Check sheet for the modelled part. Datum: model origin and axes. Units: mm. Face numbers are marked on the shaded views. A direction names the side the tool comes from. Round coordinates to 2 decimals unless told otherwise and drop trailing zeros. Order: outer loops, then holes, each group sorted by start corner. A loop starts at its lowest first (then second) coordinate and runs counter-clockwise, first axis right, second up.
```python
from build123d import *

# Parameters (mm, degrees)
F0_R     = 4.75
F1_DEPTH = 2
F2_W     = 1
F2_H     = 0.5
F3_W     = 1
F3_H     = 0.5
F4_DEPTH = 2.5
F5_R     = 0.49999
F6_R     = 0.99999


# Not quite as in the source:
# - a fillet or chamfer is up to 0.001 mm smaller than in the source, because OpenCascade refuses the exact size


with BuildPart() as f1:
    # F0 (on Top) → F1 (new body)
    with BuildSketch(Plane.XY):
        Circle(F0_R)
        with BuildLine():
            ThreePointArc((-2.6457513111, 0.75), (0, 2.75), (2.6457513111, 0.75))
            Line((2.6457513111, 0.75), (3.6457513111, 0.75))
            Line((3.6457513111, 0.75), (3.6457513111, -0.75))
            Line((3.6457513111, -0.75), (2.6457513111, -0.75))
            ThreePointArc((2.6457513111, -0.75), (0, -2.75), (-2.6457513111, -0.75))
            Line((-2.6457513111, -0.75), (-3.6457513111, -0.75))
            Line((-3.6457513111, -0.75), (-3.6457513111, 0.75))
            Line((-3.6457513111, 0.75), (-2.6457513111, 0.75))
        make_face(mode=Mode.SUBTRACT)
    extrude(amount=F1_DEPTH)

    # F2 (on face) + F3 (on face) → F4 (join)
    with BuildSketch(Plane.XZ.offset(-0.75)):
        with Locations((-3.1457513111, 1.75)):
            Rectangle(F2_W, F2_H)
        with Locations((-3.1457513111, 0.25)):
            Rectangle(F2_W, F2_H)
    with BuildSketch(Plane.XZ.offset(-0.75)):
        with Locations((3.1457513111, 0.25)):
            Rectangle(F3_W, F3_H)
        with Locations((3.1457513111, 1.75)):
            Rectangle(F3_W, F3_H)
    extrude(amount=F4_DEPTH)

    # F5 (radius 0.5 in the source; OpenCascade refuses exactly that, so slightly less here)
    f5_edges = [f1.edges().sort_by_distance(p)[0] for p in [
        (-2.645751, 0, 2),
        (2.645751, 0, 2),
        (0, 2.75, 2),
        (0, -2.75, 2),
        (0, 2.75, 0),
        (0, -2.75, 0),
        (-2.645751, 0, 0),
        (2.645751, 0, 0),
    ]]
    fillet(f5_edges, radius=F5_R)

    # F6 (radius 1 in the source; OpenCascade refuses exactly that, so slightly less here)
    f6_edges = [f1.edges().sort_by_distance(p)[0] for p in [
        (-4.75, 0, 2),
        (-4.75, 0, 0),
    ]]
    fillet(f6_edges, radius=F6_R)


solid = f1.part
```
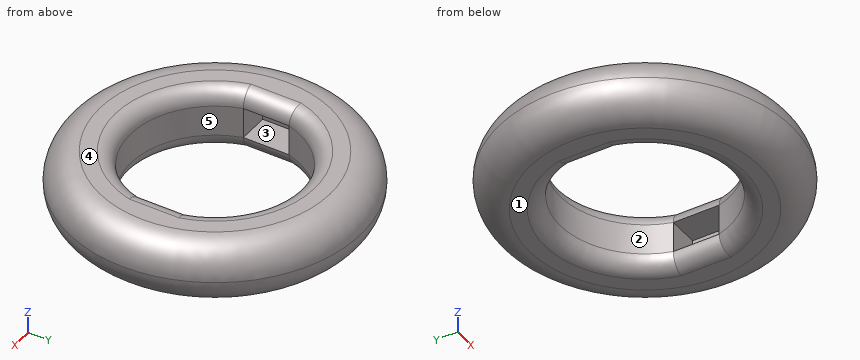
Item 1: Scan lines: line 1 along Z through (x, y) = (-3.5, -0.5); line 2 along Y through (x, z) = (-1.5, 1.7); line 3 along Y through (x, z) = (1.75, 1.5). Record each from-to range of solid material in increasing order.
Answer:
line 1: z = 0 to 0.5, 1.5 to 2
line 2: y = -4.2 to -2.35, 2.35 to 4.2
line 3: y = -4.27 to -2.12, 2.12 to 4.27
Item 2: Access from +Z, -Z, +X, -X, +Y, -Y to the whole of each face (thin tool, end or side, straight path). Record for the marked faces 3, 4 and 5.
Answer:
face 3: none
face 4: +Z, +X, -X, +Y, -Y
face 5: +Z, -Z
Item 3: Sectioned sample at C-C (z = 1.2). Record the cut outline in (x, y), and give its area (3 significant figures).
Answer:
outline: circle Ø9.46 at (0, 0); hole (-3.65, -0.75) - (-2.65, -0.75) arc R2.75 ccw to (2.65, -0.75) - (3.65, -0.75) - (3.65, 0.75) - (2.65, 0.75) arc R2.75 ccw to (-2.65, 0.75) - (-3.65, 0.75) - close
area: 43.7 mm2
Item 4: Sectioned sample at D-D (z = 0.3). Record the cut outline in (x, y), and give its area (3 significant figures).
Answer:
outline: circle Ø8.93 at (0, 0); hole (-2.69, -0.76) arc R2.79 ccw to (2.69, -0.76) - (2.69, 0.76) arc R2.79 ccw to (-2.69, 0.76) - close
area: 38.3 mm2
Item 5: Release check for a two-part mould opening along Y. For the marked faces 1 and 2 record: released by +Y, released by -Y, zero draft, split by the parting line, or undercut.
Answer:
face 1: zero draft
face 2: undercut
Item 6: Go/stop test with flat-tipped pins: P1, Ø1.1, axis at x = -3, z = 1, coming from the -Y side; P2, Ø0.8, axis at x = -3, z = 1, coming from the +Y side; P3, Ø1.1, axis at x = 3, z = 1, coming from the +Y side. Record where each tip stops, or that it passes through.
Answer:
P1: stops at y = -4.07
P2: stops at y = 3.98
P3: stops at y = 4.07
